from build123d import *


with BuildPart() as f4:
    # F4: sweep along a path in F0, F6
    with BuildLine(Plane.XY) as f4_path:
        ThreePointArc((0, 30), (-51.2132034356, 51.2132034356), (-30, 0))
        ThreePointArc((-30, 0), (-8.7867965644, -8.7867965644), (0, -30))
    with BuildLine(Plane(origin=(0, 0, 0), x_dir=(0, -1, 0), z_dir=(-1, 0, 0))) as f4_path_2:
        ThreePointArc((30, 0), (51.2132034356, -51.2132034356), (0, -30))
        ThreePointArc((0, -30), (-6.7735276417, -10.5626982962), (-24.16013062, 0.4552602768))
    # F5 (on offset) → F4 (sweep)
    with BuildSketch(Plane.XZ.offset(-30)):
        Polygon((-3.75, -6.4951905284), (7.5, 0), (-3.75, 6.4951905284), align=None)
    sweep(path=f4_path.line + f4_path_2.line)


solid = f4.part
Build history of the part. All positions in model axes, mm. A direction names the side the tool comes from. Coordinates: 2 decimals unless noted, no trailing zeros. Write each question's results on one line, items separated by ' | '. Start each with the question number.
Item 1: Wall check: probe 1 along Y at (x, z) = (-4, -21); probe 2 along Z at (x, y) = (-1.5, -19.5); probe 3 along Y at (x, z) = (-30, 3). Give the ranges that are in metal, low to high. Write a range as [from, to].
Item 2: Flat gauge pins, fed straight in: pin 1 (2 mm diameter, centred on x = -52, y = 43, fed in from +Z); pin 2 (6 mm diameter, centred on x = -56, y = 48.5, fed in from +Z); pin 3 (1.5 mm diameter, centred on x = -34.5, y = -9.5, fed in from -Z); pin 4 (22 mm diameter, centred on y = -35.5, z = -16.5, fed in from +X). Where does each tip first touch, or does it go through?
Item 3: Tool access for faces 1 (the face through (-0.55, 24.14, 0.54)), 2 (the face through (1, 30, 0)): list every direction of +Z, -Z, +X, -X, +Y, -Y with a clear straight run to the whole face (end or side of a thin tool).
Item 4: Mould opens along Y. For faces 3 (the face through (-47.9, 49.2, -0.1)), 4 (the face through (3.75, -11, -45)) say: released by +Y, released by -Y, zero draft, split by the parting line, or undercut.
Numbers:
1) probe 1: [-60.73, -56.49], [-0.78, 3.44] | probe 2: [-61.77, -54.37], [-4.55, 4.55] | probe 3: [-2.3, 3.75], [56.25, 62.3]
2) pin 1: z = 6.5 | pin 2: z = 4.96 | pin 3: through | pin 4: x = 3.75
3) face 1: +Z, +X | face 2: +Z, -Z, +X
4) face 3: undercut | face 4: zero draft
